Check sheet for the modelled part. Datum: model origin and axes. Units: mm. Face numbers are marked on the shaded views. A direction names the side the tool comes from. Coordinates: 2 decimals unless noted, no trailing zeros. Order: outer loops, then holes, each group sorted by start corner. A loop starts at its lowest first (then second) coordinate and runs counter-clockwise, first axis right, second up.
1. Cross-section at D-D (x = -112.5). Enter the section's corners in (y, z).
2. Thickness scan on line 1 (Z direction, x = -118.5, y = 8); line 2 (X direction, y = 1.75, z = 28); line 3 (Y direction, x = -109, z = 23). Record the ranges inside material, lowest first.
3. Cross-section at A-A (x = -12). Enter the section's corners in (y, z).
4. Cross-section at C-C (z = 86). Enter the section's corners in (x, y).
5. Gauge pin test, flat ends, axial feed: pin 1 Ø10 at (x, z) = (-84.5, 268) entering from +Y; pin 2 Ø3 at (y, z) = (30.5, 41.5) entering from +X; pin 3 Ø2 at (x, z) = (-64, 272) entering from +Y; pin 4 Ø4.5 at (x, z) = (-64, 28) entering from -Y. Record the tip position at first contact, or that the pin passes through.
6. Set-up check for the marked faces 4 and 5: record each of +Z, -Z, +X, -X, +Y, -Y from which the full face is reachable in a straight line by a thin tool's end or side.
7. Draft check along Z on the marked faces 1, 2 and 3. Enter one of: released by +Z, released by -Z, zero draft, split by the parting line, or undercut.
8. Cross-section at B-B (y = 46). Enter the section's corners in (x, z), then the cut area to 3 significant figures.
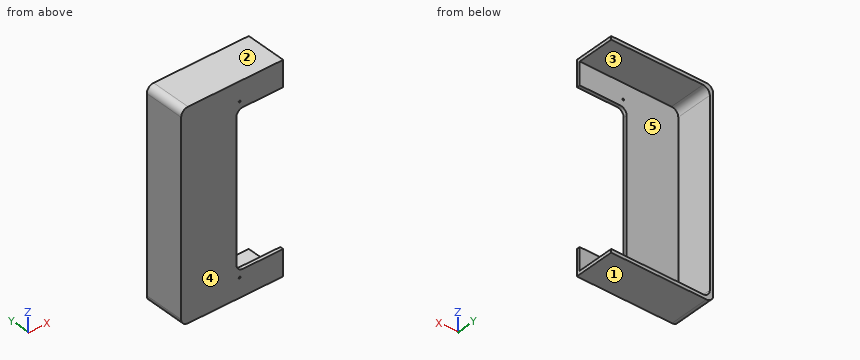
```python
from build123d import *

# Parameters (mm, degrees)
SKETCH_1_W          = 150
SKETCH_1_H          = 300
EXTRUDE_1_DEPTH     = 60
CUT_EXTRUDE_1_DEPTH = 55
SKETCH_3_W          = 69
SKETCH_3_H          = 224
CUT_EXTRUDE_2_DEPTH = 5
SKETCH_4_R          = 1.4
CUT_EXTRUDE_3_DEPTH = 5
FILLET_1_R          = 10


with BuildPart() as part:
    # 草图1 → 凸台-拉伸1 (new body)
    with BuildSketch(Plane(origin=(0, 0, 0), x_dir=(1, 0, 0), z_dir=(0, 1, 0))):
        with Locations((-75, -150)):
            Rectangle(SKETCH_1_W, SKETCH_1_H)
    extrude(amount=EXTRUDE_1_DEPTH)

    # 草图2 → 切除-拉伸1 (cut)
    with BuildSketch(Plane(origin=(0, 60, 0), x_dir=(1, 0, 0), z_dir=(0, 1, 0))):
        Polygon((-5, -5), (-145, -5), (-145, -295), (-5, -295), (0, -295), (0, -5), align=None)
    extrude(amount=-CUT_EXTRUDE_1_DEPTH, mode=Mode.SUBTRACT)

    # 草图3 → 切除-拉伸2 (cut)
    with BuildSketch(Plane(origin=(0, 5, 0), x_dir=(1, 0, 0), z_dir=(0, 1, 0))):
        with Locations((-34.5, -150)):
            Rectangle(SKETCH_3_W, SKETCH_3_H)
    extrude(amount=-CUT_EXTRUDE_2_DEPTH, mode=Mode.SUBTRACT)

    # 草图4 → 切除-拉伸3 (cut)
    with BuildSketch(Plane(origin=(0, 5, 0), x_dir=(1, 0, 0), z_dir=(0, 1, 0))):
        with Locations(Location((-64, -28, 0), (0, 0, 270))):
            Circle(SKETCH_4_R)
        with Locations(Location((-64, -272, 0), (0, 0, 90))):
            Circle(SKETCH_4_R)
    extrude(amount=-CUT_EXTRUDE_3_DEPTH, mode=Mode.SUBTRACT)

    # 圆角1
    fillet_1_edges = [part.edges().sort_by_distance(p)[0] for p in [
        (-145, 32.5, 5),
        (-145, 32.5, 295),
        (-69, 2.5, 38),
        (-69, 2.5, 262),
        (-150, 30, 300),
        (-150, 30, 0),
    ]]
    fillet(fillet_1_edges, radius=FILLET_1_R)


solid = part.part
```
Data:
1. outline: (0, 0) - (60, 0) - (60, 5) - (5, 5) - (5, 295) - (60, 295) - (60, 300) - (0, 300) - close
2. line 1: z = 0 to 5, 295 to 300
2. line 2: x = -150 to -65.4, -62.6 to 0
2. line 3: y = 0 to 5
3. outline: (0, 0) - (60, 0) - (60, 5) - (5, 5) - (5, 38) - (0, 38) - close; (0, 262) - (5, 262) - (5, 295) - (60, 295) - (60, 300) - (0, 300) - close
4. outline: (-150, 0) - (-69, 0) - (-69, 5) - (-145, 5) - (-145, 60) - (-150, 60) - close
5. pin 1: stops at y = 5
5. pin 2: stops at x = -145
5. pin 3: passes through
5. pin 4: stops at y = 0
6. face 4: +Z, -Z, +X, -X, -Y
6. face 5: +X, +Y
7. face 1: released by -Z
7. face 2: released by +Z
7. face 3: undercut
8. outline: (-150, 10) arc R10 ccw to (-140, 0) - (0, 0) - (0, 5) - (-135, 5) arc R10 cw to (-145, 15) - (-145, 285) arc R10 cw to (-135, 295) - (0, 295) - (0, 300) - (-140, 300) arc R10 ccw to (-150, 290) - close
8. area: 2,950 mm2
